Design review of the part shown in the three views and the two pictorial views. Dimensions are in mm from the part's minimum x, y and z. Round coordinates to 2 decimals unless told otherwise and drop trailing zeros. Loops run counter-clockwise (first coordinate to the right, second up) from the corner with the lowest first, then second, coordinate; pieces in that order, holes last.
1. Clearance check with flat-ended pins moving along their axes: pin 1 Ø3.5 at (x, y) = (15.74, 46.49) entering from +Z; pin 2 Ø1 at (y, z) = (10.5, 1) entering from -X. State where each tip first meets the part, or that it passes through.
2. Consider section C-C on z = 1.7. State the section outline as (x, y) points (1 decimal).
3. Consider section B-B on y = 27. State the section outline as (x, z) points.
4. Consider section A-A on x = 27. State the section outline as (y, z) points, then the cut area to 3 significant figures.
5. To check wall thickness, follow line 1 along Y through (x, z) = (37.5, 2.05) (1 decimal); line 2 along Y through (x, z) = (38, 1.9); line 3 along X through (y, z) = (7, 1.25). State the ranges of each line that lie inside material, in increasing order.
6. Draft analysis for pull direction Y (two halves, no side actions). For the marked faces 1, 2 and 3, state which applies: released by +Y, released by -Y, zero draft, split by the parting line, or undercut.
7. Consider section D-D on x = 49.51. State the section outline as (y, z) points.
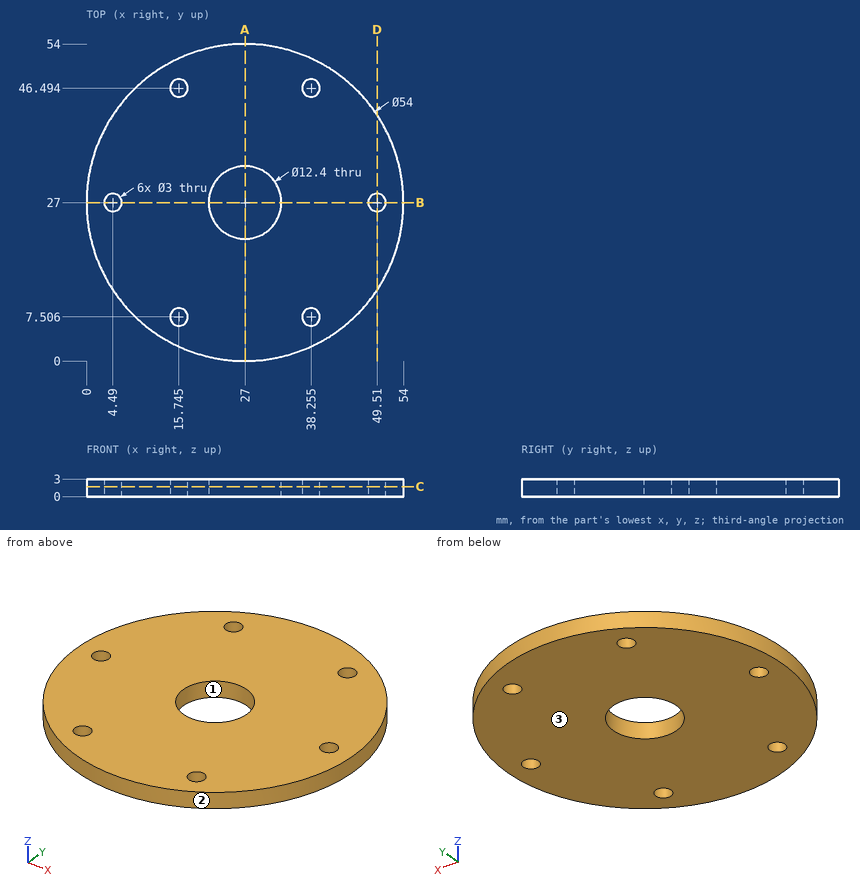
Resolved:
1. pin 1: stops at z = 3
1. pin 2: stops at x = 5.25
2. outline: circle Ø54 at (27, 27); hole circle Ø3 at (4.5, 27); hole circle Ø3 at (15.7, 7.5); hole circle Ø3 at (15.7, 46.5); hole circle Ø12.4 at (27, 27); hole circle Ø3 at (38.3, 7.5); hole circle Ø3 at (38.3, 46.5); hole circle Ø3 at (49.5, 27)
3. outline: (0, 0) - (2.99, 0) - (2.99, 3) - (0, 3) - close; (5.99, 0) - (20.8, 0) - (20.8, 3) - (5.99, 3) - close; (33.2, 0) - (48.01, 0) - (48.01, 3) - (33.2, 3) - close; (51.01, 0) - (54, 0) - (54, 3) - (51.01, 3) - close
4. outline: (0, 0) - (20.8, 0) - (20.8, 3) - (0, 3) - close; (33.2, 0) - (54, 0) - (54, 3) - (33.2, 3) - close
4. area: 125 mm2
5. line 1: y = 2.1 to 6.2, 8.8 to 45.2, 47.8 to 51.9
5. line 2: y = 2.34 to 6.03, 8.98 to 45.02, 47.97 to 51.66
5. line 3: x = 8.86 to 14.33, 17.16 to 36.84, 39.67 to 45.14
6. face 1: undercut
6. face 2: split by the parting line
6. face 3: zero draft
7. outline: (12.09, 0) - (25.5, 0) - (25.5, 3) - (12.09, 3) - close; (28.5, 0) - (41.91, 0) - (41.91, 3) - (28.5, 3) - close
